Work out the finished part from the listing and answer in its coordinate system (mm). A direction names the side the tool comes from. Round coordinates to 2 decimals unless told otherwise and drop trailing zeros. Order: outer loops, then holes, each group sorted by start corner. A loop starts at its lowest first (then second) coordinate and runs counter-clockwise, first axis right, second up. Notation, with made-up numbers: (56, 72.25) - (75, 72.25) arc R29 cw to (75, 101.25) - close; hole circle Ø7 at (-4.75, -11.5). An arc over 180 degrees is marked (long way). Answer in a Markdown table with one row per item.
from build123d import *

# Parameters (mm, degrees)
SKETCH2_W           = 300
SKETCH2_H           = 7.5
BOSS_EXTRUDE1_DEPTH = 30
SKETCH3_W           = 3
SKETCH3_H           = 30
BOSS_EXTRUDE2_DEPTH = 5
SKETCH4_W           = 3
SKETCH4_H           = 30
BOSS_EXTRUDE3_DEPTH = 66
SKETCH5_W           = 300
SKETCH5_H           = 30
BOSS_EXTRUDE4_DEPTH = 29.5
SKETCH6_W           = 290
SKETCH6_H           = 20
CUT_EXTRUDE1_DEPTH  = 306.68909869


with BuildPart() as part:
    # Sketch2 → Boss-Extrude1 (new body)
    with BuildSketch(Plane.XY):
        with Locations((137.761363636, -0.5625)):
            Rectangle(SKETCH2_W, SKETCH2_H)
    extrude(amount=BOSS_EXTRUDE1_DEPTH)

    # Sketch3 → Boss-Extrude2 (add)
    with BuildSketch(Plane.XZ.offset(4.3125)):
        with Locations((231.761363636, 15)):
            Rectangle(SKETCH3_W, SKETCH3_H)
        with Locations((43.761363636, 15)):
            Rectangle(SKETCH3_W, SKETCH3_H)
    extrude(amount=BOSS_EXTRUDE2_DEPTH)

    # Sketch4 → Boss-Extrude3 (add)
    with BuildSketch(Plane(origin=(0, 3.1875, 0), x_dir=(1, 0, 0), z_dir=(0, 1, 0))):
        with Locations((171.761363636, -15)):
            Rectangle(SKETCH4_W, SKETCH4_H)
        with Locations((103.761363636, -15)):
            Rectangle(SKETCH4_W, SKETCH4_H)
    extrude(amount=BOSS_EXTRUDE3_DEPTH)

    # Sketch5 → Boss-Extrude4 (add)
    with BuildSketch(Plane(origin=(0, 69.1875, 0), x_dir=(1, 0, 0), z_dir=(0, 1, 0))):
        with Locations((137.761363636, -15)):
            Rectangle(SKETCH5_W, SKETCH5_H)
    extrude(amount=BOSS_EXTRUDE4_DEPTH)

    # Sketch6 → Cut-Extrude1 (cut, through all)
    with BuildSketch(Plane(origin=(0, 0, 0), x_dir=(-1, 0, 0), z_dir=(0, 0, -1))):
        with Locations((-137.761363636, 83.6875)):
            Rectangle(SKETCH6_W, SKETCH6_H)
    extrude(amount=-CUT_EXTRUDE1_DEPTH, mode=Mode.SUBTRACT)


solid = part.part
1) The mould has two halves that part along X. Classify faces 1 (the face through (-7.239, 84, 15)), 2 (the face through (260, -4.312, 15)), 3 (the face through (102.261, 36, 15)): released by +X, released by -X, zero draft, split by the parting line, or undercut.
Filled in:
| item | result |
|---|---|
| face 1 | undercut |
| face 2 | zero draft |
| face 3 | released by -X |
2) Find section B-B, the plane z = 17.25. Give the vertices of the cut face in (x, y).
Filled in:
| item | result |
|---|---|
| outline | (-12.24, -4.31) - (42.26, -4.31) - (42.26, -9.31) - (45.26, -9.31) - (45.26, -4.31) - (230.26, -4.31) - (230.26, -9.31) - (233.26, -9.31) - (233.26, -4.31) - (287.76, -4.31) - (287.76, 3.19) - (173.26, 3.19) - (173.26, 69.19) - (287.76, 69.19) - (287.76, 98.69) - (-12.24, 98.69) - (-12.24, 69.19) - (102.26, 69.19) - (102.26, 3.19) - (-12.24, 3.19) - close; hole (-7.24, 73.69) - (282.76, 73.69) - (282.76, 93.69) - (-7.24, 93.69) - close; hole (105.26, 3.19) - (170.26, 3.19) - (170.26, 69.19) - (105.26, 69.19) - close |
3) Find section D-D, the plane y = 54. Give the vertices of the cut face in (x, z).
Filled in:
| item | result |
|---|---|
| outline | (102.26, 0) - (105.26, 0) - (105.26, 30) - (102.26, 30) - close; (170.26, 0) - (173.26, 0) - (173.26, 30) - (170.26, 30) - close |
4) Which of the six approach directions +Z, -Z, +X, -X, +Y, -Y give full straight-line access (tool end or side, diameter ignored) to faces 4 (the face through (230, 3.188, 15)), 5 (the face through (44, 3.188, 15)), 6 (the face through (230.261, -7, 15)), 7 (the face through (140, 73.688, 15)), 8 (the face through (287.761, 84, 15))?
Filled in:
| item | result |
|---|---|
| face 4 | +Z, -Z, +X |
| face 5 | +Z, -Z, -X |
| face 6 | +Z, -Z, -Y |
| face 7 | +Z, -Z |
| face 8 | +Z, -Z, +X, +Y, -Y |
5) Find section A-A, the plane y = 85.5. Give the vertices of the cut face in (x, z).
Filled in:
| item | result |
|---|---|
| outline | (-12.24, 0) - (-7.24, 0) - (-7.24, 30) - (-12.24, 30) - close; (282.76, 0) - (287.76, 0) - (287.76, 30) - (282.76, 30) - close |
6) Each of these flat-tipped pins is pushed along its axis until it touches: pin 1 (4 mm diameter, centred on x = 90, z = 12.5, fed in from -Y); pin 2 (2.5 mm diameter, centred on y = -7, z = 16.5, fed in from -X); pin 3 (9 mm diameter, centred on y = 26, z = 19.5, fed in from +X). Where does it stop, or does it pass through?
Filled in:
| item | result |
|---|---|
| pin 1 | stops at y = -4.31 |
| pin 2 | stops at x = 42.26 |
| pin 3 | stops at x = 173.26 |
7) Find section C-C, the plane x = 134.5. Give the vertices of the cut face in (y, z).
Filled in:
| item | result |
|---|---|
| outline | (-4.31, 0) - (3.19, 0) - (3.19, 30) - (-4.31, 30) - close; (69.19, 0) - (73.69, 0) - (73.69, 30) - (69.19, 30) - close; (93.69, 0) - (98.69, 0) - (98.69, 30) - (93.69, 30) - close |
8) Find the intervals of material crossed by probe 1 along Y at (x, z) = (264, 16); probe 2 along X at (y, z) = (34.5, 7.5); probe 3 along X at (y, z) = (82.5, 2.75), in increasing order. Write a range as from..to.
Filled in:
| item | result |
|---|---|
| probe 1 | y = -4.31..3.19, 69.19..73.69, 93.69..98.69 |
| probe 2 | x = 102.26..105.26, 170.26..173.26 |
| probe 3 | x = -12.24..-7.24, 282.76..287.76 |
